Part model, mm, in its own coordinate system. Face numbers are marked on the shaded views. Coordinates: 2 decimals unless noted, no trailing zeros. Write each loop counter-clockwise with the first axis right and the second up, starting at its lowest first coordinate (ties: lowest second). Pieces come first, ordered by that corner, then holes. Notation, with made-up numbers: M 23,79.25 L 42,79.25 A19 ccw 42,97.25 Z; hole C 36.5,-1 d8. An arc over 180 degrees is marked long. Use a Markdown table: item, result. Add a question column.
Q1. Wall check: L1, parallel to Z at x = 5, y = 25. Give the ranges that are in metal, low to high. Write a range as from..to.
Q2. Slice it at B-B on x = -15. Write the cut outline in (y, z).
Q3. Slice it at A-A on z = 10. Write the cut outline in (x, y).
Q4. Mould opens along Y. For the marked faces 1, 2 and 3 say: released by +Y, released by -Y, zero draft, split by the parting line, or undercut.
Q5. Slice it at C-C on y = 22.5. Write the cut outline in (x, z), then the cut area to 3 significant figures.
Q6. Pin check, flat tips, straight feed: pin 1 Ø6 at (x, z) = (-21, 15.5) entering from +Y; pin 2 Ø9 at (x, y) = (-17.21, 18) entering from -Z. Stop position of each tip, or through.
Q7. Slice it at D-D on y = 18. Write the cut outline in (x, z).
from build123d import *

# Parameters (mm, degrees)
SKETCH_1_W          = 46
SKETCH_1_H          = 34
EXTRUDE_1_DEPTH     = 2
SKETCH_2_W          = 46
SKETCH_2_H          = 2
EXTRUDE_2_DEPTH     = 30
SKETCH_3_R          = 5.5
CUT_EXTRUDE_1_DEPTH = 2
CUT_EXTRUDE_2_DEPTH = 2


with BuildPart() as part:
    # 草图1 → 凸台-拉伸1 (new body)
    with BuildSketch(Plane.XY):
        with Locations((-7.206275861, 17)):
            Rectangle(SKETCH_1_W, SKETCH_1_H)
    extrude(amount=EXTRUDE_1_DEPTH)

    # 草图2 → 凸台-拉伸2 (add)
    with BuildSketch(Plane.XY.offset(2)):
        with Locations((-7.206275861, 1)):
            Rectangle(SKETCH_2_W, SKETCH_2_H)
    extrude(amount=EXTRUDE_2_DEPTH)

    # 草图3 → 切除-拉伸1 (cut)
    with BuildSketch(Plane.XY.offset(2)):
        with Locations((-17.206275861, 18)):
            Circle(SKETCH_3_R)
    extrude(amount=-CUT_EXTRUDE_1_DEPTH, mode=Mode.SUBTRACT)

    # 草图4 → 切除-拉伸2 (cut)
    with BuildSketch(Plane(origin=(0, 2, 0), x_dir=(1, 0, 0), z_dir=(0, 1, 0))):
        with BuildLine():
            Line((-24.235699599, -7.328343443), (-24.235699599, -28.539953108))
            ThreePointArc((-24.235699599, -28.539953108), (-22.841637624, -29.934015083), (-21.447575649, -28.539953108))
            Line((-21.447575649, -28.539953108), (-21.447575649, -7.328343443))
            ThreePointArc((-21.447575649, -7.328343443), (-22.841637624, -5.934281468), (-24.235699599, -7.328343443))
        make_face()
        with BuildLine():
            Line((7.035023927, -7.328343443), (7.035023927, -28.539953108))
            ThreePointArc((7.035023927, -28.539953108), (8.429085903, -29.934015083), (9.823147878, -28.539953108))
            Line((9.823147878, -28.539953108), (9.823147878, -7.328343443))
            ThreePointArc((9.823147878, -7.328343443), (8.429085903, -5.934281468), (7.035023927, -7.328343443))
        make_face()
    extrude(amount=-CUT_EXTRUDE_2_DEPTH, mode=Mode.SUBTRACT)


solid = part.part
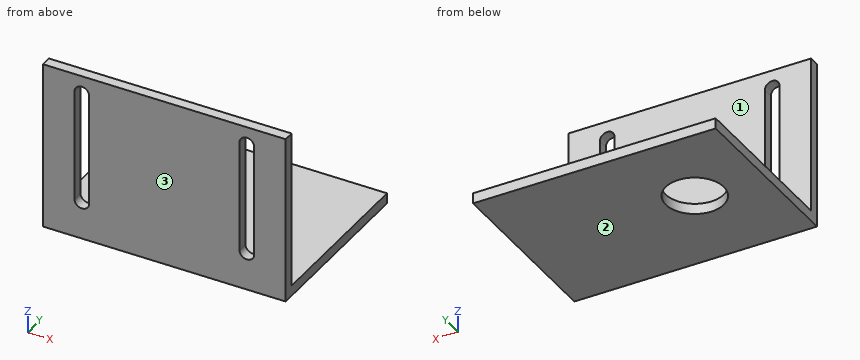
Recorded:
| question | item | result |
|---|---|---|
| 1 | L1 | 0..2 |
| 2 | outline | M 0,0 L 12.96,0 L 12.96,2 L 2,2 L 2,32 L 0,32 Z; M 23.04,0 L 34,0 L 34,2 L 23.04,2 Z |
| 3 | outline | M -30.21,0 L -24.24,0 L -24.24,2 L -30.21,2 Z; M -21.45,0 L 7.04,0 L 7.04,2 L -21.45,2 Z; M 9.82,0 L 15.79,0 L 15.79,2 L 9.82,2 Z |
| 4 | face 1 | released by +Y |
| 4 | face 2 | zero draft |
| 4 | face 3 | released by -Y |
| 5 | outline | M -30.21,0 L -20.37,0 L -20.37,2 L -30.21,2 Z; M -14.04,0 L 15.79,0 L 15.79,2 L -14.04,2 Z |
| 5 | area | 79.4 mm² |
| 6 | pin 1 | y = 2 |
| 6 | pin 2 | through |
| 7 | outline | M -30.21,0 L -22.71,0 L -22.71,2 L -30.21,2 Z; M -11.71,0 L 15.79,0 L 15.79,2 L -11.71,2 Z |
